Design review of the part built by this model. Coordinates are the model's own, in mm. Give positions to 0.01 mm unless a question says otherwise; leave off trailing zeros. Write each loop counter-clockwise with the first axis right and the second up, starting at its lowest first coordinate (ties: lowest second). Pieces come first, ordered by that corner, then holes.
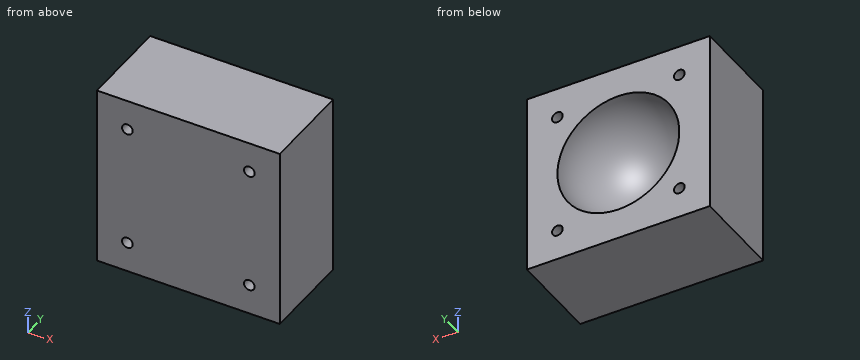
```python
from build123d import *

# Parameters (mm, degrees)
SKETCH1_W           = 60
SKETCH1_H           = 60
BOSS_EXTRUDE1_DEPTH = 30
CUT_REVOLVE1_ANGLE  = 180
SKETCH3_R           = 1.75
CUT_EXTRUDE1_DEPTH  = 30


with BuildPart() as part:
    # Sketch1 → Boss-Extrude1 (new body)
    with BuildSketch(Plane(origin=(0, 0, 0), x_dir=(1, 0, 0), z_dir=(0, 1, 0))):
        Rectangle(SKETCH1_W, SKETCH1_H)
    extrude(amount=BOSS_EXTRUDE1_DEPTH)

    # Sketch2 → Cut-Revolve1 (revolve, cut)
    with BuildSketch(Plane(origin=(0, 30, 0), x_dir=(1, 0, 0), z_dir=(0, 1, 0))):
        with BuildLine():
            Line((0, 20), (0, -20))
            ThreePointArc((0, -20), (20, 0), (0, 20))
        make_face()
    revolve(axis=Axis((0, 30, -20), (0, 0, -1)), revolution_arc=CUT_REVOLVE1_ANGLE, mode=Mode.SUBTRACT)

    # Sketch3 → Cut-Extrude1 (cut)
    with BuildSketch(Plane(origin=(0, 30, 0), x_dir=(1, 0, 0), z_dir=(0, 1, 0))):
        with Locations(Location((-20, 20, 0), (0, 0, 270))):
            Circle(SKETCH3_R)
        with Locations(Location((-20, -20, 0), (0, 0, 270))):
            Circle(SKETCH3_R)
        with Locations(Location((20, 20, 0), (0, 0, 270))):
            Circle(SKETCH3_R)
        with Locations(Location((20, -20, 0), (0, 0, 270))):
            Circle(SKETCH3_R)
    extrude(amount=-CUT_EXTRUDE1_DEPTH, mode=Mode.SUBTRACT)


solid = part.part
```
(1) Consider section C-C, the plane x = -9. Give the boundary of the cut face in (y, z).
Resolved:
outline: (0, -30) - (30, -30) - (30, -17.86) arc R17.86 cw to (30, 17.86) - (30, 30) - (0, 30) - close
(2) Consider section A-A, the plane z = 16. Give the boundary of the cut face in (x, y), then the cut area to 3 significant figures.
Resolved:
outline: (-30, 0) - (30, 0) - (30, 30) - (12, 30) arc R12 cw to (-12, 30) - (-30, 30) - close
area: 1,570 mm2
(3) To check wall thickness, follow L1, parallel to X at y = 16.75, z = -20; L2, parallel to X at y = 23, z = -19; L3, parallel to X at y = 21, z = 13.5. State the ranges of each line that lie inside material, in increasing order.
Resolved:
L1: x = -30 to -21.75, -18.25 to 18.25, 21.75 to 30
L2: x = -30 to -21.44, -18.56 to 18.56, 21.44 to 30
L3: x = -30 to -11.69, 11.69 to 30
(4) Consider section B-B, the plane z = -21. Give the boundary of the cut face in (x, y).
Resolved:
outline: (-30, 0) - (-21.44, 0) - (-21.44, 30) - (-30, 30) - close; (-18.56, 0) - (18.56, 0) - (18.56, 30) - (-18.56, 30) - close; (21.44, 0) - (30, 0) - (30, 30) - (21.44, 30) - close
